Geometry: final body of the model. Coordinates: model frame, mm. A direction names the side the tool comes from. Round coordinates to 2 decimals unless told otherwise and drop trailing zeros. Write each loop counter-clockwise with the first axis right and the second up, starting at its lowest first coordinate (ties: lowest second). Pieces come first, ordered by that corner, then holes. Notation, with made-up numbers: (29, 58) -> (59, 58) arc R14 ccw to (59, 77) -> close; hole circle Ø9 at (-34, 39). An arc over 180 degrees is marked (long way). Use one line per item in the form item = value. Start each with the question number.
1. Pin query (flat end, axial travel): pin 1 Ø8 at (y, z) = (24, -4.5) entering from +X; pin 2 Ø1 at (x, z) = (7.5, 3) entering from +Y. Return the tip coordinate at first contact, or that it passes through.
2. Draft query along Z for faces 6 (the face through (-9.4, 15.9, -7.5)), 7 (the face through (9.76, 34.1, 6.64)), 8 (the face through (9.74, 33.433, -0.846)). Return one class per face: pulls with the +Z half, pulls with the -Z half, needs draft (parallel to the pull), parting line crosses it, or undercut.
3. Cut plane A-A, the plane z = 3.75. Return the cut outline in (x, y), plus the area to 3 significant figures.
4. Line query: L1, parallel to X at y = 19, z = 0.5; L2, parallel to Y at x = -4.5, z = 2; L3, parallel to Y at x = -9.25, z = 0. Output: solid intervals per line, ascending.
5. Reachability of faces 1 (the face through (9.76, 34.1, -6.64)), 2 (the face through (-2, 4, -2)), 3 (the face through (9, 16, 0)), 4 (the face through (1.802, 0.493, 5.723)), 5 (the face through (-10.5, 16, 0)) from +Z, -Z, +X, -X, +Y, -Y: full face, straight path, thin tool, end or side. Return the list, or none.
6. Cut plane D-D, the plane y = 25.5. Return the cut outline in (x, z), plus the area to 3 significant figures.
7. Cut plane C-C, the plane z = 0. Return the cut outline in (x, y), plus the area to 3 significant figures.
8. Cut plane B-B, the plane x = 0. Return the cut outline in (y, z).
```python
from build123d import *

# Parameters (mm, degrees)
CROQUIS1_R              = 6
SALIENTE_EXTRUIR1_DEPTH = 1
CROQUIS2_R              = 2.5
SALIENTE_EXTRUIR2_DEPTH = 3
CROQUIS3_W              = 21
CROQUIS3_H              = 15
SALIENTE_EXTRUIR3_DEPTH = 1
CROQUIS4_W              = 1.5
CROQUIS4_H              = 15
SALIENTE_EXTRUIR4_DEPTH = 30
CROQUIS5_R              = 6.5
CORTAR_EXTRUIR1_DEPTH   = 34
REDONDEO1_R             = 3


with BuildPart() as part:
    # Croquis1 → Saliente-Extruir1 (new body)
    with BuildSketch(Plane(origin=(0, 0, 0), x_dir=(1, 0, 0), z_dir=(0, 1, 0))):
        with Locations(Location((0, 0, 0), (0, 0, 270))):
            Circle(CROQUIS1_R)
    extrude(amount=SALIENTE_EXTRUIR1_DEPTH)

    # Croquis2 → Saliente-Extruir2 (add)
    with BuildSketch(Plane(origin=(0, 1, 0), x_dir=(1, 0, 0), z_dir=(0, 1, 0))):
        with Locations(Location((0, 0, 0), (0, 0, 270))):
            Circle(CROQUIS2_R)
    extrude(amount=SALIENTE_EXTRUIR2_DEPTH)

    # Croquis3 → Saliente-Extruir3 (add)
    with BuildSketch(Plane(origin=(0, 4, 0), x_dir=(1, 0, 0), z_dir=(0, 1, 0))):
        Rectangle(CROQUIS3_W, CROQUIS3_H)
    extrude(amount=SALIENTE_EXTRUIR3_DEPTH)

    # Croquis4 → Saliente-Extruir4 (add)
    with BuildSketch(Plane(origin=(0, 5, 0), x_dir=(1, 0, 0), z_dir=(0, 1, 0))):
        with Locations((-9.75, 0)):
            Rectangle(CROQUIS4_W, CROQUIS4_H)
        with Locations((9.75, 0)):
            Rectangle(CROQUIS4_W, CROQUIS4_H)
    extrude(amount=SALIENTE_EXTRUIR4_DEPTH)

    # Croquis5 → Cortar-Extruir1 (cut)
    with BuildSketch(Plane.ZY.offset(10.5)):
        with Locations((0, 26.988393785)):
            Circle(CROQUIS5_R)
    extrude(amount=-CORTAR_EXTRUIR1_DEPTH, mode=Mode.SUBTRACT)

    # Redondeo1
    redondeo1_edges = [part.edges().sort_by_distance(p)[0] for p in [
        (-9.75, 35, 7.5),
        (-9.75, 35, -7.5),
        (9.75, 35, -7.5),
        (9.75, 35, 7.5),
    ]]
    fillet(redondeo1_edges, radius=REDONDEO1_R)


solid = part.part
```
Outcome:
q1.pin_1 = 10.5
q1.pin_2 = 5
q2.face_6 = pulls with the -Z half
q2.face_7 = pulls with the +Z half
q2.face_8 = undercut
q3.outline = (-10.5, 4) -> (10.5, 4) -> (10.5, 21.68) -> (9, 21.68) -> (9, 5) -> (-9, 5) -> (-9, 21.68) -> (-10.5, 21.68) -> close; (-10.5, 32.3) -> (-9, 32.3) -> (-9, 35) -> (-10.5, 35) -> close; (-4.68, 0) -> (4.68, 0) -> (4.68, 1) -> (-4.68, 1) -> close; (9, 32.3) -> (10.5, 32.3) -> (10.5, 35) -> (9, 35) -> close
q3.area = 88.5 mm^2
q4.L1 = -10.5 to -9, 9 to 10.5
q4.L2 = 0 to 1, 4 to 5
q4.L3 = 4 to 20.49, 33.49 to 35
q5.face_1 = -Z, +X, -X, +Y
q5.face_2 = none
q5.face_3 = +Z, -Z, +Y
q5.face_4 = -Y
q5.face_5 = +Z, -Z, -X, +Y, -Y
q6.outline = (-10.5, -7.5) -> (-9, -7.5) -> (-9, -6.33) -> (-10.5, -6.33) -> close; (-10.5, 6.33) -> (-9, 6.33) -> (-9, 7.5) -> (-10.5, 7.5) -> close; (9, -7.5) -> (10.5, -7.5) -> (10.5, -6.33) -> (9, -6.33) -> close; (9, 6.33) -> (10.5, 6.33) -> (10.5, 7.5) -> (9, 7.5) -> close
q6.area = 7.04 mm^2
q7.outline = (-10.5, 4) -> (-2.5, 4) -> (-2.5, 1) -> (-6, 1) -> (-6, 0) -> (6, 0) -> (6, 1) -> (2.5, 1) -> (2.5, 4) -> (10.5, 4) -> (10.5, 20.49) -> (9, 20.49) -> (9, 5) -> (-9, 5) -> (-9, 20.49) -> (-10.5, 20.49) -> close; (-10.5, 33.49) -> (-9, 33.49) -> (-9, 35) -> (-10.5, 35) -> close; (9, 33.49) -> (10.5, 33.49) -> (10.5, 35) -> (9, 35) -> close
q7.area = 99.0 mm^2
q8.outline = (0, -6) -> (1, -6) -> (1, -2.5) -> (4, -2.5) -> (4, -7.5) -> (5, -7.5) -> (5, 7.5) -> (4, 7.5) -> (4, 2.5) -> (1, 2.5) -> (1, 6) -> (0, 6) -> close
